For this review, take the finished solid that the model builds, in its own axes (mm). A direction names the side the tool comes from. Round coordinates to 2 decimals unless told otherwise and drop trailing zeros. Order: outer loops, then holes, each group sorted by start corner. A loop starts at its lowest first (then second) coordinate and runs counter-clockwise, first axis right, second up. Notation, with made-up numbers: (22.5, 74.25) - (72.5, 74.25) arc R22 ccw to (72.5, 90.25) - close; hole circle Ø3 at (48.5, 32.25). An arc over 180 degrees is marked (long way). One line per question, with ' | ' between items.
```python
from build123d import *

# Parameters (mm, degrees)
SKETCH1_W           = 38
SKETCH1_H           = 38
BOSS_EXTRUDE1_DEPTH = 2
SKETCH2_W           = 38
SKETCH2_H           = 2
BOSS_EXTRUDE2_DEPTH = 38
SKETCH3_R           = 3
CUT_EXTRUDE1_DEPTH  = 10
SKETCH4_R           = 3
CUT_EXTRUDE2_DEPTH  = 10


with BuildPart() as part:
    # Sketch1 → Boss-Extrude1 (new body)
    with BuildSketch(Plane(origin=(0, 0, 0), x_dir=(1, 0, 0), z_dir=(0, 1, 0))):
        with Locations((-13.081650622, 15.738235294)):
            Rectangle(SKETCH1_W, SKETCH1_H)
    extrude(amount=BOSS_EXTRUDE1_DEPTH)

    # Sketch2 → Boss-Extrude2 (add)
    with BuildSketch(Plane(origin=(0, 2, 0), x_dir=(1, 0, 0), z_dir=(0, 1, 0))):
        with Locations((-13.081650622, 33.738235294)):
            Rectangle(SKETCH2_W, SKETCH2_H)
    extrude(amount=BOSS_EXTRUDE2_DEPTH)

    # Sketch3 → Cut-Extrude1 (cut)
    with BuildSketch(Plane.XY.offset(-32.738235294)):
        with Locations((-13.081650622, 30)):
            Circle(SKETCH3_R)
        with Locations((-13.081650622, 12)):
            Circle(SKETCH3_R)
    extrude(amount=-CUT_EXTRUDE1_DEPTH, mode=Mode.SUBTRACT)

    # Sketch4 → Cut-Extrude2 (cut)
    with BuildSketch(Plane(origin=(0, 2, 0), x_dir=(1, 0, 0), z_dir=(0, 1, 0))):
        with Locations(Location((-13.081650622, 5.738235294, 0), (0, 0, 270))):
            Circle(SKETCH4_R)
        with Locations(Location((-13.081650622, 23.738235294, 0), (0, 0, 270))):
            Circle(SKETCH4_R)
    extrude(amount=-CUT_EXTRUDE2_DEPTH, mode=Mode.SUBTRACT)


solid = part.part
```
(1) We need section A-A on y = 30. State the section outline as (x, z) points.
Output values:
outline: (-32.08, -34.74) - (-16.08, -34.74) - (-16.08, -32.74) - (-32.08, -32.74) - close; (-10.08, -34.74) - (5.92, -34.74) - (5.92, -32.74) - (-10.08, -32.74) - close
(2) Insertion check: pin 1 (8 mm diameter, centred on x = -13.08, y = 12, fed in from -Z); pin 2 (5 mm diameter, centred on x = -15, z = -16, fed in from +Y); pin 3 (3 mm diameter, centred on x = -9, y = 24.5, fed in from +Z). Each pin has a flat end and moves straight along its axis. Give the tip position at first contact, or say it passes through.
Output values:
pin 1: z = -34.74 | pin 2: y = 2 | pin 3: z = -32.74
(3) We need section D-D on y = 23. State the section outline as (x, z) points.
Output values:
outline: (-32.08, -34.74) - (5.92, -34.74) - (5.92, -32.74) - (-32.08, -32.74) - close
(4) We need section B-B on z = -25. State the section outline as (x, y) points, plus the area to 3 significant figures.
Output values:
outline: (-32.08, 0) - (-15.8, 0) - (-15.8, 2) - (-32.08, 2) - close; (-10.36, 0) - (5.92, 0) - (5.92, 2) - (-10.36, 2) - close | area: 65.1 mm^2
(5) Mouldability with a two-part tool opening along Y and no side actions: class faces 1 (the flat face through (-13, 0, -16)), 2 (the cylindrical face through (-12.181, 1.014, -20.877)), 3 (the cylindrical face through (-16.08, 30.13, -33.72)) as released by +Y, released by -Y, zero draft, split by the parting line, or undercut.
Output values:
face 1: released by -Y | face 2: zero draft | face 3: undercut
(6) We need section C-C on x = -27. State the section outline as (y, z) points.
Output values:
outline: (0, -34.74) - (40, -34.74) - (40, -32.74) - (2, -32.74) - (2, 3.26) - (0, 3.26) - close
(7) For probe 1 along Z at (x, y) = (-20, 33.5); probe 2 along Y at (x, z) = (-23.5, -25), list the stretches that pass through material, from the lowest coordinate up. Write a range as [from, to].
Output values:
probe 1: [-34.74, -32.74] | probe 2: [0, 2]
(8) For faces 4 (the flat face through (5.918, 11, -34)), 5 (the flat face through (-13, 21, -32.738)), list the 3-axis set-ups (+Z, -Z, +X, -X, +Y, -Y) from which the entire face can be reached by the end or side of a thin tool; tool diameter is ignored.
Output values:
face 4: +Z, -Z, +X, +Y, -Y | face 5: +Z, +X, -X, +Y
